Verification items for this drawing (mm, ordinates from the low corner). A direction names the side the tool comes from. Coordinates: 2 decimals unless noted, no trailing zeros. Write each loop counter-clockwise with the first axis right and the second up, starting at its lowest first coordinate (ties: lowest second). Pieces come first, ordered by that corner, then holes. Notation, with made-up numbers: (-25.5, 39) -> (21.5, 39) arc R30 cw to (21.5, 75) -> close; hole circle Ø3 at (62, 32). An arc over 180 degrees is marked (long way). One line per question, with ' | ' between items.
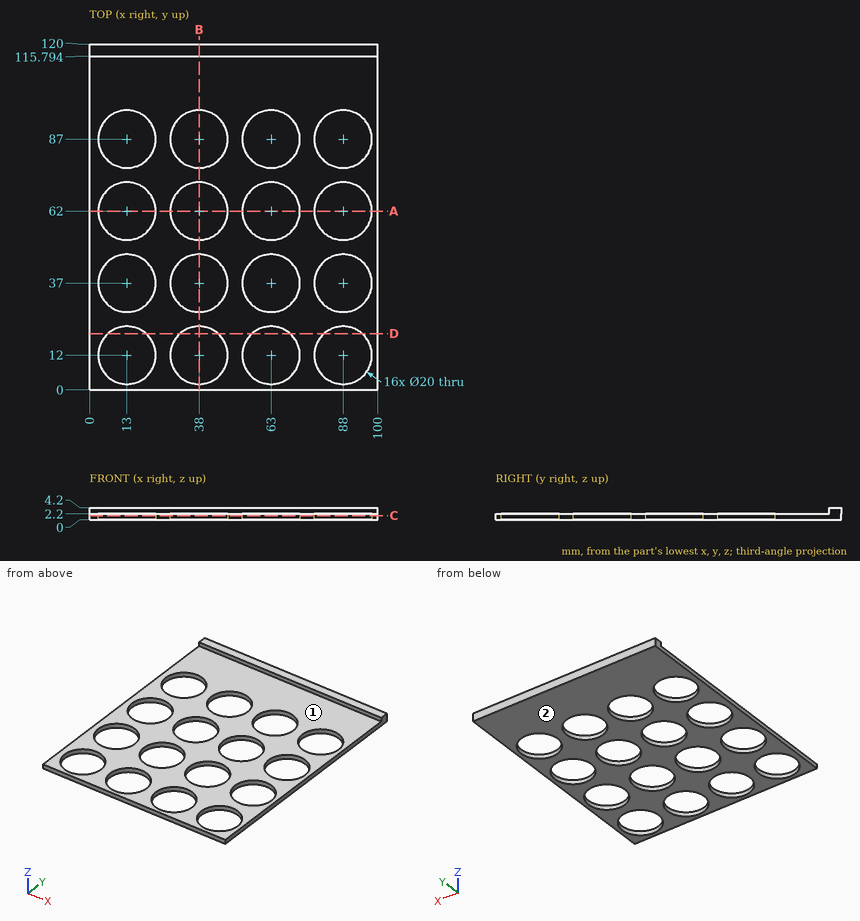
(1) Tool access check on the marked faces 1 and 2. Record the directions out of +Z, -Z, +X, -X, +Y, -Y that give a thin tool (end or side, any length) a straight path to the whole face; none if there is none.
Answers below:
face 1: +Z, +X, -X, -Y | face 2: -Z, +X, -X, +Y, -Y
(2) Cross-section at B-B (x = 38). Record the cut outline in (y, z) (1 decimal).
Answers below:
outline: (0, 0) -> (2, 0) -> (2, 2.2) -> (0, 2.2) -> close; (22, 0) -> (27, 0) -> (27, 2.2) -> (22, 2.2) -> close; (47, 0) -> (52, 0) -> (52, 2.2) -> (47, 2.2) -> close; (72, 0) -> (77, 0) -> (77, 2.2) -> (72, 2.2) -> close; (97, 0) -> (120, 0) -> (120, 4.2) -> (115.8, 4.2) -> (115.8, 2.2) -> (97, 2.2) -> close
(3) Material ranges on line 1 (Y direction, x = 88, z = 1.3); line 2 (Y direction, x = 80, z = 0.85); line 3 (X direction, y = 10, z = 1.7), recorded low to high.
Answers below:
line 1: y = 0 to 2, 22 to 27, 47 to 52, 72 to 77, 97 to 120 | line 2: y = 0 to 6, 18 to 31, 43 to 56, 68 to 81, 93 to 120 | line 3: x = 0 to 3.2, 22.8 to 28.2, 47.8 to 53.2, 72.8 to 78.2, 97.8 to 100
(4) Cross-section at D-D (y = 19.5). Record the cut outline in (x, z) (1 decimal).
Answers below:
outline: (0, 0) -> (6.4, 0) -> (6.4, 2.2) -> (0, 2.2) -> close; (19.6, 0) -> (31.4, 0) -> (31.4, 2.2) -> (19.6, 2.2) -> close; (44.6, 0) -> (56.4, 0) -> (56.4, 2.2) -> (44.6, 2.2) -> close; (69.6, 0) -> (81.4, 0) -> (81.4, 2.2) -> (69.6, 2.2) -> close; (94.6, 0) -> (100, 0) -> (100, 2.2) -> (94.6, 2.2) -> close
(5) Cross-section at A-A (y = 62). Record the cut outline in (x, z).
Answers below:
outline: (0, 0) -> (3, 0) -> (3, 2.2) -> (0, 2.2) -> close; (23, 0) -> (28, 0) -> (28, 2.2) -> (23, 2.2) -> close; (48, 0) -> (53, 0) -> (53, 2.2) -> (48, 2.2) -> close; (73, 0) -> (78, 0) -> (78, 2.2) -> (73, 2.2) -> close; (98, 0) -> (100, 0) -> (100, 2.2) -> (98, 2.2) -> close
(6) Cross-section at C-C (z = 1.45). Count the separate pieces of the cut face and the enclosed holes in it, plus the area to 3 significant figures.
Answers below:
separate pieces: 1 | enclosed holes: 16 | area: 6,970 mm²
(7) Depth check by flat-ended pin: P1, Ø23, axis at x = 88, y = 37, coming from the +Z side; P2, Ø12, axis at x = 38, y = 62, coming from the +Z side; P3, Ø1, axis at x = 49.5, z = 3.5, coming from the -Y side. Enter the tip coordinate at first touch or a pass-through.
Answers below:
P1: stops at z = 2.2 | P2: passes through | P3: stops at y = 115.79
